```python
from build123d import *

# Parameters (mm, degrees)
BOSS_EXTRUDE1_DEPTH = 110
FILLET1_R           = 60
FILLET3_R           = 30
FILLET4_R           = 10
SKETCH2_R           = 1.75
CUT_EXTRUDE1_DEPTH  = 250


with BuildPart() as part:
    # Sketch1 → Boss-Extrude1 (new body)
    with BuildSketch(Plane.XY):
        Polygon((0, 0), (110, 0), (110, -250), (0, -250), (0, -230), (90, -230), (90, -20), (0, -20), align=None)
    extrude(amount=BOSS_EXTRUDE1_DEPTH)

    # Fillet1
    fillet1_edges = [part.edges().sort_by_distance(p)[0] for p in [
        (110, 0, 55),
        (110, -250, 55),
    ]]
    fillet(fillet1_edges, radius=FILLET1_R)

    # Fillet3
    fillet3_edges = [part.edges().sort_by_distance(p)[0] for p in [
        (90, -230, 55),
        (90, -20, 55),
    ]]
    fillet(fillet3_edges, radius=FILLET3_R)

    # Fillet4
    fillet4_edges = [part.edges().sort_by_distance(p)[0] for p in [
        (0, -10, 0),
        (0, 0, 55),
        (0, -250, 55),
        (0, -230, 55),
        (0, -20, 55),
        (0, -240, 110),
        (25, 0, 0),
        (25, 0, 110),
        (25, -250, 110),
        (110, -125, 0),
        (92.426406871, -232.426406871, 0),
        (92.426406871, -17.573593129, 0),
        (110, -125, 110),
        (92.426406871, -232.426406871, 110),
        (92.426406871, -17.573593129, 110),
        (0, -10, 110),
        (25, -250, 0),
        (0, -240, 0),
    ]]
    fillet(fillet4_edges, radius=FILLET4_R - 0.0001)  # a hair under: the kernel refuses the full size

    # Sketch2 → Cut-Extrude1 (cut)
    with BuildSketch(Plane.ZY.offset(-90)):
        with Locations((56.069625953, -89.440859908)):
            Circle(SKETCH2_R)
        with Locations((79.452311855, -129.940859908)):
            Circle(SKETCH2_R)
        with Locations((32.686940051, -129.940859908)):
            Circle(SKETCH2_R)
    extrude(amount=-CUT_EXTRUDE1_DEPTH, mode=Mode.SUBTRACT)


solid = part.part
```
Geometry check sheet. Reference: the model listing, model coordinates, mm. A direction names the side the tool comes from. Give positions to 0.01 mm unless a question says otherwise; leave off trailing zeros. Write each loop counter-clockwise with the first axis right and the second up, starting at its lowest first coordinate (ties: lowest second). Pieces come first, ordered by that corner, then holes. Notation, with made-up numbers: (4.25, -24) - (31.25, -24) arc R26 ccw to (31.25, -10) - close; hole circle Ø5 at (5.25, 53). An arc over 180 degrees is marked (long way). Use a Markdown table: item, result.
Q1. Draft check along Y on faces 3 (the face through (92, -124, 0)), 4 (the face through (90, -126, 54)), 5 (the face through (35, -20, 54)), 6 (the face through (30, 0, 54)). Enter one of: pulls with the +Y half, pulls with the -Y half, needs draft (parallel to the pull), parting line crosses it, or undercut.
Computed:
| item | result |
|---|---|
| face 3 | needs draft |
| face 4 | undercut |
| face 5 | undercut |
| face 6 | pulls with the +Y half |
Q2. Go/stop test with flat-tipped pins: P1, Ø2, axis at y = -89.44, z = 56.07, coming from the +X side; P2, Ø3, axis at y = -86.5, z = 22.5, coming from the -X side; P3, Ø1, axis at x = 60.5, z = 22.5, coming from the +Y side; P4, Ø1.5, axis at x = 88, z = 88.5, coming from the +Y side. Record where each tip stops, or that it passes through.
Computed:
| item | result |
|---|---|
| P1 | passes through |
| P2 | stops at x = 90 |
| P3 | stops at y = -0.84 |
| P4 | stops at y = -12.96 |
Q3. Thickness scan on L1, parallel to Y at x = 44.5, z = 17; L2, parallel to Y at x = 7, z = 89.5; L3, parallel to X at y = -120, z = 26.5. Record the ranges inside material, lowest first. Write a range as [from, to].
Computed:
| item | result |
|---|---|
| L1 | y = [-250, -230], [-20, 0] |
| L2 | y = [-249.54, -230.46], [-19.54, -0.46] |
| L3 | x = [90, 110] |
Q4. Section check C-C, the plane y = -105.5. Enter the section's corners in (x, z), then the cut area to 3 significant figures.
Computed:
| item | result |
|---|---|
| outline | (90, 0) - (100, 0) arc R10 ccw to (110, 10) - (110, 100) arc R10 ccw to (100, 110) - (90, 110) - close |
| area | 2,160 mm² |
Q5. Section check A-A, the plane x = 29.5. Enter the section's corners in (y, z), then the cut area to 3 significant figures.
Computed:
| item | result |
|---|---|
| outline | (-250, 10) arc R10 ccw to (-240, 0) - (-230, 0) - (-230, 110) - (-240, 110) arc R10 ccw to (-250, 100) - close; (-20, 0) - (-10, 0) arc R10 ccw to (0, 10) - (0, 100) arc R10 ccw to (-10, 110) - (-20, 110) - close |
| area | 4,310 mm² |
Q6. Section check D-D, the plane z = 103. Enter the section's corners in (x, y), then the cut area to 3 significant figures.
Computed:
| item | result |
|---|---|
| outline | (0.46, -240) arc R9.54 ccw to (10, -249.54) - (50, -249.54) arc R59.54 ccw to (109.54, -190) - (109.54, -60) arc R59.54 ccw to (50, -0.46) - (10, -0.46) arc R9.54 ccw to (0.46, -10) - (0.46, -13) arc R10 ccw to (10, -20) - (60, -20) arc R30 cw to (90, -50) - (90, -200) arc R30 cw to (60, -230) - (10, -230) arc R10 ccw to (0.46, -237) - close |
| area | 7,160 mm² |
Q7. Set-up check for faces 1 (the face through (92.89, -231.96, 55.63)), 2 (the face through (35, -230, 54)): record each of +Z, -Z, +X, -X, +Y, -Y from which the full face is reachable in a straight line by a thin tool's end or side.
Computed:
| item | result |
|---|---|
| face 1 | +Z, -Z, +X, -Y |
| face 2 | +Z, -Z, -X |
